Can you work these out from the model? Positions are in its coordinate system, mm. Face numbers are marked on the shaded views. A direction names the side the tool comes from. Coordinates: 2 decimals unless noted, no trailing zeros. Write each loop counter-clockwise with the first axis right and the second up, starting at its lowest first coordinate (ties: lowest second). Pieces come first, ordered by that corner, then holes. Notation, with made-up numbers: (68, 35) - (112, 35) arc R27 cw to (112, 64) - close; hole circle Ø11 at (54.25, 14). An arc over 180 degrees is marked (long way). Use one line per item in the form item = value. Start each with the question number.
(1) If I drill on probe 1 along Y at (x, z) = (0, 1.2); probe 2 along X at (y, z) = (0, 2.2); probe 3 along Y at (x, z) = (0, 0.95), over which ranges is the centre line in solid material (lowest first)? Write a range as from..to.
(2) For pin 1 Ø2.5 at (x, y) = (0, 0) entering from +Z; pin 2 Ø3 at (x, z) = (-7.5, 2.5) entering from -Y, each with a flat end and sliding along its axis, tell me the tip position at first contact or that it passes through.
(3) If we section it at B-B on z = 2.5: Please give me the cut outline in (x, y), then the cut area to 3 significant figures.
(4) On a 3-axis mill with a long thin cutter (end or side, diameter ignored), from which of +Z, -Z, +X, -X, +Y, -Y can I reach the whole of each face in a straight line? I mean the marked faces 4 and 5. Say none if no direction works.
(5) Thinking about a two-plate mould opening in X: for the marked faces 1, 2 and 3, which applies, pulls with the +X half, pulls with the -X half, needs draft (parallel to the pull), parting line crosses it, or undercut?
(6) If we section it at A-A on z = -0.55: Please give me the cut outline in (x, y), then the cut area to 3 significant figures.
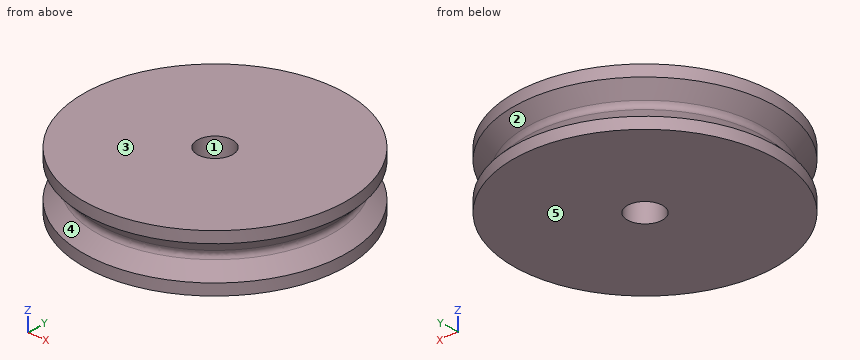
```python
from build123d import *

# Parameters (mm, degrees)
F0_R        = 11.5
F0_R_2      = 1.55
F2_DEPTH    = 4
F2_FACE_R   = 11.5
F2_FACE_R_2 = 1.55
F4_DEPTH    = 1
F5_R        = 0.5


with BuildPart() as f2:
    # F0 (on Top) → F2 (new body)
    with BuildSketch(Plane.XY):
        Circle(F0_R)
        Circle(F0_R_2, mode=Mode.SUBTRACT)
    extrude(amount=F2_DEPTH)

    # F1 (on Front) → F3 (revolve, cut)
    with BuildSketch(Plane.XZ):
        Polygon((-11.5, 3), (-11.5, 0), (-10, 1.5), align=None)
    revolve(axis=Axis((0, 0, 1.929782), (0, 0, 1)), mode=Mode.SUBTRACT)

    # F2_face (on face) → F4 (join)
    with BuildSketch(Plane(origin=(0, 0, 0), x_dir=(1, 0, 0), z_dir=(0, 0, -1))):
        Circle(F2_FACE_R)
        Circle(F2_FACE_R_2, mode=Mode.SUBTRACT)
    extrude(amount=F4_DEPTH)

    # F5
    f5_edges = [f2.edges().sort_by_distance(p)[0] for p in [
        (10, 0, 1.5),
    ]]
    fillet(f5_edges, radius=F5_R)


solid = f2.part
```
Reported:
q1.probe_1 = -10.31..-1.55, 1.55..10.31
q1.probe_2 = -10.7..-1.55, 1.55..10.7
q1.probe_3 = -10.55..-1.55, 1.55..10.55
q2.pin_1 = through
q2.pin_2 = -9.76
q3.outline = circle Ø22 at (0, 0); hole circle Ø3.1 at (0, 0)
q3.area = 373 mm2
q4.face_4 = none
q4.face_5 = -Z, +X, -X, +Y, -Y
q5.face_1 = undercut
q5.face_2 = parting line crosses it
q5.face_3 = needs draft
q6.outline = circle Ø23 at (0, 0); hole circle Ø3.1 at (0, 0)
q6.area = 408 mm2
